```python
from build123d import *

# Parameters (mm, degrees)
SKETCH_1_R                 = 18.3
SKETCH_1_R_2               = 13
SKETCH_1_R_3               = 6
SKETCH_1_R_4               = 1.5
SKETCH_1_R_5               = 3
EXTRUDE_2_DEPTH            = 21.5
CUT_EXTRUDE_8_DEPTH        = 1
SKETCH_1_10_R              = 1.5
CUT_EXTRUDE_9_DEPTH        = 5
EXTRUDE_START              = -6
SKETCH_1_11_R              = 6
SKETCH_1_11_R_2            = 3
EXTRUDE_3_DEPTH            = 6
EXTRUDE_START_2            = -19.8
SKETCH_1_12_R              = 3
EXTRUDE_4_DEPTH            = 19.8
CUT_EXTRUDE_10_DEPTH       = 11.5
SKETCH_4_R                 = 16.4
EXTRUDE_5_DEPTH            = 23
SKETCH_5_R                 = 0.75
EXTRUDE_6_DEPTH            = 6
SKETCH_5_3_R               = 15.5
SKETCH_5_3_R_2             = 0.75
SKETCH_5_3_R_3             = 3.5
EXTRUDE_7_DEPTH            = 3
CUT_EXTRUDE_11_OUTLINE_R   = 15.5
CUT_EXTRUDE_11_OUTLINE_R_2 = 0.75
CUT_EXTRUDE_11_OUTLINE_R_3 = 3.5
CUT_EXTRUDE_11_DEPTH       = 2
SKETCH_6_R                 = 7
EXTRUDE_8_DEPTH            = 4
SKETCH_6_3_W               = 16
SKETCH_6_3_H               = 4
EXTRUDE_9_DEPTH            = 6
SKETCH_7_R                 = 0.5
CUT_EXTRUDE_12_DEPTH       = 0.5
SKETCH_8_W                 = 16.4
SKETCH_8_H                 = 4.4
CUT_EXTRUDE_13_DEPTH       = 4.5
SKETCH_9_R                 = 0.4
EXTRUDE_10_DEPTH           = 4


# Read off the part's stored shape, not the designer's step: 切除-拉伸11
with BuildPart() as part:
    # 草图1 → 凸台-拉伸2 (new body)
    # profile 1 of 15: a face of its own
    with BuildSketch(Plane(origin=(0, 0, 0), x_dir=(1, 0, 0), z_dir=(0, 1, 0))):
        with Locations(Location((0, 0, 0), (0, 0, 270))):
            Circle(SKETCH_1_R)
        Circle(SKETCH_1_R_2, mode=Mode.SUBTRACT)
        with Locations((7.3, 0)):
            Circle(SKETCH_1_R_3, mode=Mode.SUBTRACT)
        with Locations((-13.423393759, 7.75)):
            Circle(SKETCH_1_R_4, mode=Mode.SUBTRACT)
        with Locations((-13.423393759, -7.75)):
            Circle(SKETCH_1_R_4, mode=Mode.SUBTRACT)
        with Locations((0, -15.5)):
            Circle(SKETCH_1_R_4, mode=Mode.SUBTRACT)
        with Locations((13.423393759, -7.75)):
            Circle(SKETCH_1_R_4, mode=Mode.SUBTRACT)
        with Locations((13.423393759, 7.75)):
            Circle(SKETCH_1_R_4, mode=Mode.SUBTRACT)
        with Locations((0, 15.5)):
            Circle(SKETCH_1_R_4, mode=Mode.SUBTRACT)
    # profile 2 of 15: a face of its own
    with BuildSketch(Plane(origin=(0, 0, 0), x_dir=(1, 0, 0), z_dir=(0, 1, 0))):
        Circle(SKETCH_1_R_2)
    # profile 3 of 15: a face of its own
    with BuildSketch(Plane(origin=(0, 0, 0), x_dir=(1, 0, 0), z_dir=(0, 1, 0))):
        with Locations((7.3, 0)):
            Circle(SKETCH_1_R_3)
    # profile 4 of 15: a face of its own
    with BuildSketch(Plane(origin=(0, 0, 0), x_dir=(1, 0, 0), z_dir=(0, 1, 0))):
        with Locations((0, 15.5)):
            Circle(SKETCH_1_R_4)
    # profile 5 of 15: a face of its own
    with BuildSketch(Plane(origin=(0, 0, 0), x_dir=(1, 0, 0), z_dir=(0, 1, 0))):
        with Locations((-13.423393759, 7.75)):
            Circle(SKETCH_1_R_4)
    # profile 6 of 15: a face of its own
    with BuildSketch(Plane(origin=(0, 0, 0), x_dir=(1, 0, 0), z_dir=(0, 1, 0))):
        with Locations((-13.423393759, -7.75)):
            Circle(SKETCH_1_R_4)
    # profile 7 of 15: a face of its own
    with BuildSketch(Plane(origin=(0, 0, 0), x_dir=(1, 0, 0), z_dir=(0, 1, 0))):
        with Locations((0, -15.5)):
            Circle(SKETCH_1_R_4)
    # profile 8 of 15: a face of its own
    with BuildSketch(Plane(origin=(0, 0, 0), x_dir=(1, 0, 0), z_dir=(0, 1, 0))):
        with Locations((13.423393759, -7.75)):
            Circle(SKETCH_1_R_4)
    # profile 9 of 15: a face of its own
    with BuildSketch(Plane(origin=(0, 0, 0), x_dir=(1, 0, 0), z_dir=(0, 1, 0))):
        with Locations((13.423393759, 7.75)):
            Circle(SKETCH_1_R_4)
    # profile 10 of 15: a face of its own
    with BuildSketch(Plane(origin=(0, 0, 0), x_dir=(1, 0, 0), z_dir=(0, 1, 0))):
        with Locations((7.3, 0)):
            Circle(SKETCH_1_R_5)
    # profile 11 of 15: a face of its own
    with BuildSketch(Plane(origin=(0, 0, 0), x_dir=(1, 0, 0), z_dir=(0, 1, 0))):
        with Locations((7.3, 0)):
            Circle(SKETCH_1_R_3)
    # profile 12 of 15: a face of its own
    with BuildSketch(Plane(origin=(0, 0, 0), x_dir=(1, 0, 0), z_dir=(0, 1, 0))):
        Circle(SKETCH_1_R_2)
    # profile 13 of 15: a face of its own
    with BuildSketch(Plane(origin=(0, 0, 0), x_dir=(1, 0, 0), z_dir=(0, 1, 0))):
        with Locations((7.3, 0)):
            Circle(SKETCH_1_R_5)
    # profile 14 of 15: a face of its own
    with BuildSketch(Plane(origin=(0, 0, 0), x_dir=(1, 0, 0), z_dir=(0, 1, 0))):
        Circle(SKETCH_1_R_2)
    # profile 15 of 15: a face of its own
    with BuildSketch(Plane(origin=(0, 0, 0), x_dir=(1, 0, 0), z_dir=(0, 1, 0))):
        with Locations((7.3, 0)):
            Circle(SKETCH_1_R_3)
    extrude(amount=EXTRUDE_2_DEPTH)

    # 草图1<9> → 切除-拉伸8 (cut)
    with BuildSketch(Plane(origin=(0, 0, 0), x_dir=(1, 0, 0), z_dir=(0, 1, 0))):
        with BuildLine():
            ThreePointArc((12.759589041, -2.488551286), (1.3, 0), (12.759589041, 2.488551286))
            ThreePointArc((12.759589041, 2.488551286), (-13, 0), (12.759589041, -2.488551286))
        make_face()
    extrude(amount=CUT_EXTRUDE_8_DEPTH, mode=Mode.SUBTRACT)

    # 草图1<10> → 切除-拉伸9 (cut)
    with BuildSketch(Plane(origin=(0, 0, 0), x_dir=(1, 0, 0), z_dir=(0, 1, 0))):
        with Locations(Location((13.423393759, 7.75, 0), (0, 0, 270))):
            Circle(SKETCH_1_10_R)
        with Locations(Location((0, 15.5, 0), (0, 0, 270))):
            Circle(SKETCH_1_10_R)
        with Locations(Location((-13.423393759, 7.75, 0), (0, 0, 270))):
            Circle(SKETCH_1_10_R)
        with Locations(Location((-13.423393759, -7.75, 0), (0, 0, 270))):
            Circle(SKETCH_1_10_R)
        with Locations(Location((0, -15.5, 0), (0, 0, 270))):
            Circle(SKETCH_1_10_R)
        with Locations(Location((13.423393759, -7.75, 0), (0, 0, 270))):
            Circle(SKETCH_1_10_R)
    extrude(amount=CUT_EXTRUDE_9_DEPTH, mode=Mode.SUBTRACT)

    # 草图1<11> → 凸台-拉伸3 (add)
    with BuildSketch(Plane(origin=(0, 0, 0), x_dir=(1, 0, 0), z_dir=(0, 1, 0)).offset(EXTRUDE_START)):
        with Locations(Location((7.3, 0, 0), (0, 0, 24.504112001))):
            Circle(SKETCH_1_11_R)
        with Locations(Location((7.3, 0, 0), (0, 0, 270))):
            Circle(SKETCH_1_11_R_2, mode=Mode.SUBTRACT)
    extrude(amount=EXTRUDE_3_DEPTH)

    # 草图1<12> → 凸台-拉伸4 (add)
    with BuildSketch(Plane(origin=(0, 0, 0), x_dir=(1, 0, 0), z_dir=(0, 1, 0)).offset(EXTRUDE_START_2)):
        with Locations(Location((7.3, 0, 0), (0, 0, 270))):
            Circle(SKETCH_1_12_R)
    extrude(amount=EXTRUDE_4_DEPTH)

    # 草图3 → 切除-拉伸10 (cut)
    with BuildSketch(Plane.XZ.offset(19.8)):
        with BuildLine():
            Line((4.8, -1.658312395), (4.8, 1.658312395))
            ThreePointArc((4.8, 1.658312395), (4.3, 0), (4.8, -1.658312395))
        make_face()
    extrude(amount=-CUT_EXTRUDE_10_DEPTH, mode=Mode.SUBTRACT)

    # 草图4 → 凸台-拉伸5 (add)
    with BuildSketch(Plane(origin=(0, 21.5, 0), x_dir=(1, 0, 0), z_dir=(0, 1, 0))):
        with Locations(Location((0, 0, 0), (0, 0, 270))):
            Circle(SKETCH_4_R)
    extrude(amount=EXTRUDE_5_DEPTH)

    # 草图5 → 凸台-拉伸6 (add)
    with BuildSketch(Plane(origin=(0, 44.5, 0), x_dir=(1, 0, 0), z_dir=(0, 1, 0))):
        with Locations(Location((-10, 0, 0), (0, 0, 270))):
            Circle(SKETCH_5_R)
        with Locations(Location((10, 0, 0), (0, 0, 90))):
            Circle(SKETCH_5_R)
    extrude(amount=EXTRUDE_6_DEPTH)

    # 草图5<3> → 凸台-拉伸7 (add)
    # profile 1 of 2: a face of its own
    with BuildSketch(Plane(origin=(0, 44.5, 0), x_dir=(1, 0, 0), z_dir=(0, 1, 0))):
        with Locations(Location((0, 0, 0), (0, 0, 270))):
            Circle(SKETCH_5_3_R)
        with Locations(Location((10, 0, 0), (0, 0, 90))):
            Circle(SKETCH_5_3_R_2, mode=Mode.SUBTRACT)
        Circle(SKETCH_5_3_R_3, mode=Mode.SUBTRACT)
        with Locations(Location((-10, 0, 0), (0, 0, 270))):
            Circle(SKETCH_5_3_R_2, mode=Mode.SUBTRACT)
    # profile 2 of 2: a face of its own
    with BuildSketch(Plane(origin=(0, 44.5, 0), x_dir=(1, 0, 0), z_dir=(0, 1, 0))):
        Circle(SKETCH_5_3_R_3)
    extrude(amount=EXTRUDE_7_DEPTH)

    # 切除-拉伸11 outline → 切除-拉伸11 (cut)
    with BuildSketch(Plane(origin=(0, 44.5, 0), x_dir=(1, 0, 0), z_dir=(0, 1, 0))):
        Circle(CUT_EXTRUDE_11_OUTLINE_R)
        with Locations((-10, 0)):
            Circle(CUT_EXTRUDE_11_OUTLINE_R_2, mode=Mode.SUBTRACT)
        Circle(CUT_EXTRUDE_11_OUTLINE_R_3, mode=Mode.SUBTRACT)
        with Locations((10, 0)):
            Circle(CUT_EXTRUDE_11_OUTLINE_R_2, mode=Mode.SUBTRACT)
    extrude(amount=CUT_EXTRUDE_11_DEPTH, mode=Mode.SUBTRACT)

    # 草图6 → 凸台-拉伸8 (add)
    with BuildSketch(Plane(origin=(0, 47.5, 0), x_dir=(1, 0, 0), z_dir=(0, 1, 0))):
        with Locations(Location((0, 0, 0), (0, 0, 270))):
            Circle(SKETCH_6_R)
    extrude(amount=EXTRUDE_8_DEPTH)

    # 草图6<3> → 凸台-拉伸9 (add)
    with BuildSketch(Plane(origin=(0, 47.5, 0), x_dir=(1, 0, 0), z_dir=(0, 1, 0))):
        with Locations((0, 10.619429464)):
            Rectangle(SKETCH_6_3_W, SKETCH_6_3_H)
        Polygon((-8, 12.619429464), (-9, 12.619429464), (-9, 7.619429464), (9, 7.619429464), (9, 12.619429464), (8, 12.619429464), (8, 8.619429464), (-8, 8.619429464), align=None)
    extrude(amount=EXTRUDE_9_DEPTH)

    # 草图7 → 切除-拉伸12 (cut)
    with BuildSketch(Plane(origin=(0, 51.5, 0), x_dir=(1, 0, 0), z_dir=(0, 1, 0))):
        with Locations(Location((0, 0, 0), (0, 0, 270))):
            Circle(SKETCH_7_R)
    extrude(amount=-CUT_EXTRUDE_12_DEPTH, mode=Mode.SUBTRACT)

    # 草图8 → 切除-拉伸13 (cut)
    with BuildSketch(Plane(origin=(0, 0, -12.619429464), x_dir=(-1, 0, 0), z_dir=(0, 0, -1))):
        with Locations((0, 50.5)):
            Rectangle(SKETCH_8_W, SKETCH_8_H)
    extrude(amount=-CUT_EXTRUDE_13_DEPTH, mode=Mode.SUBTRACT)

    # 草图9 → 凸台-拉伸10 (add)
    with BuildSketch(Plane(origin=(0, 0, -8.119429464), x_dir=(-1, 0, 0), z_dir=(0, 0, -1))):
        with Locations((-6.35, 50.5)):
            Circle(SKETCH_9_R)
        with Locations((-3.81, 50.5)):
            Circle(SKETCH_9_R)
        with Locations((-1.27, 50.5)):
            Circle(SKETCH_9_R)
        with Locations((1.27, 50.5)):
            Circle(SKETCH_9_R)
        with Locations((3.81, 50.5)):
            Circle(SKETCH_9_R)
        with Locations((6.35, 50.5)):
            Circle(SKETCH_9_R)
    extrude(amount=EXTRUDE_10_DEPTH)


solid = part.part
```
Can you work these out from the model? Positions are in its coordinate system, mm. A direction names the side the tool comes from. Coordinates: 2 decimals unless noted, no trailing zeros. Loops run counter-clockwise (first coordinate to the right, second up) from the corner with the lowest first, then second, coordinate; pieces in that order, holes last. Notation, with made-up numbers: M -34.5,58.25 L -23.5,58.25 A25 ccw -23.5,89.25 Z; hole C 54,89 d11. An arc over 180 degrees is marked long. Put each result on its own line as item: value. Start each with the question number.
(1) Imagine slicing it at A-A on z = 7.75. List the corners of the cut face in (x, y) for me, and give its area (3 significant figures).
(2) Which directions (+Z, -Z, +X, -X, +Y, -Y) give clear straight access to the entire face, cutting with the end or side of a thin tool? Please do faces 1 (the face through (0, 51.5, 1)), 2 (the face through (0, 48, -12.619)), 3 (the face through (-8.2, 50, -10)), 4 (the face through (-6.834, 49.472, -1.517)), 5 (the face through (11.96, 2.46, -8.08)).
(3) Will these pins go through, and if not, where does the flat tip stop? pin 1 Ø1.5 at (y, z) = (38, 9) entering from -X; pin 2 Ø1.8 at (x, y) = (3, 49) entering from +Z; pin 3 Ø4 at (y, z) = (52, -11.5) entering from +X; pin 4 Ø18.5 at (x, z) = (-3.5, 4.5) entering from -Y.
(4) Imagine slicing it at D-D on y = -4. List the corners of the cut face in (x, z) for me, and give its area (3 significant figures).
(5) Imagine slicing it at C-C on x = -10. List the corners of the cut face in (y, z) for me, and give its area (3 significant figures).
(6) Imagine slicing it at B-B on y = 9. List the corners of the cut face in (x, z) for me.
(7) I need wall thicknesses on probe 1 along X at (y, z) = (51.1, 0); probe 2 along Y at (x, z) = (-12, -7.5); probe 3 along Y at (x, z) = (-10, -3.5). Which ranges of each line are inside material? Lowest first, please.
(8) We'd pull the mould along Z, two halves only. Please class faces 6 (the face through (-12.99, 0.49, -0.54)), 7 (the face through (4.656, 46.993, 14.784)), 8 (the face through (4, 44.5, 0)): +Z half, -Z half, draft (parallel to the pull), parting line (faces both ways), or undercut.
Worked answers:
1. outline: M -16.58,0 L -14.92,0 L -14.92,5 L -11.92,5 L -11.92,0 L -10.44,0 L -10.44,1 L 10.44,1 L 10.44,0 L 11.92,0 L 11.92,5 L 14.92,5 L 14.92,0 L 16.58,0 L 16.58,21.5 L 14.45,21.5 L 14.45,44.5 L -14.45,44.5 L -14.45,21.5 L -16.58,21.5 Z; M -13.42,46.5 L 13.42,46.5 L 13.42,47.5 L -13.42,47.5 Z
1. area: 1,350 mm2
2. face 1: +Z, +X, -X, +Y
2. face 2: -Z, +X, -X, +Y
2. face 3: -Z
2. face 4: +Y
2. face 5: -Y
3. pin 1: stops at x = -14.17
3. pin 2: stops at z = 6.68
3. pin 3: stops at x = 9
3. pin 4: stops at y = -19.8
4. outline: C 7.3,0 d12
4. area: 113 mm2
5. outline: M 0,-15.33 L 21.5,-15.33 L 21.5,-13 L 44.5,-13 L 44.5,-0.75 L 46.5,-0.75 L 46.5,-11.84 L 47.5,-11.84 L 47.5,-0.75 L 50.5,-0.75 L 50.5,0.75 L 47.5,0.75 L 47.5,11.84 L 46.5,11.84 L 46.5,0.75 L 44.5,0.75 L 44.5,13 L 21.5,13 L 21.5,15.33 L 0,15.33 L 0,8.31 L 1,8.31 L 1,-8.31 L 0,-8.31 Z
5. area: 1,270 mm2
6. outline: C 0,0 d36.6
7. probe 1: x = -7 to -0.5, 0.5 to 7
7. probe 2: y = 5 to 44.5, 46.5 to 47.5
7. probe 3: y = 1 to 44.5, 46.5 to 47.5
8. face 6: undercut
8. face 7: parting line
8. face 8: draft
